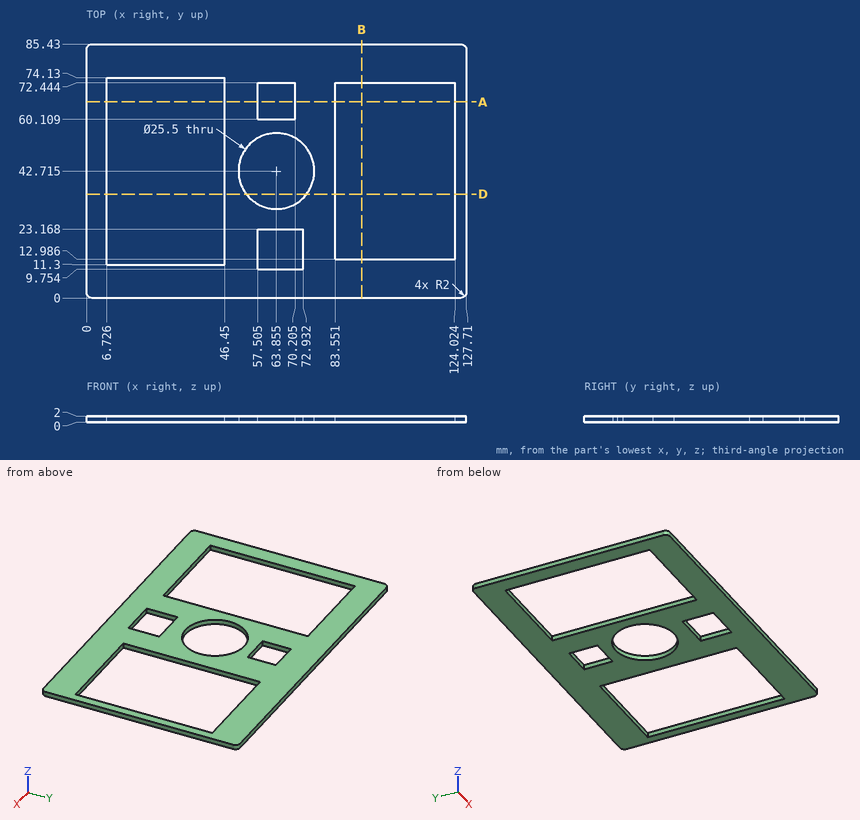
Geometry: see drawing. Coordinates: mm, zero at the bounding-box minimum. Coordinates: 2 decimals unless noted, no trailing zeros. Loops run counter-clockwise (first coordinate to the right, second up) from the corner with the lowest first, then second, coordinate; pieces in that order, holes last. Notation, with made-up numbers: (-39.5, 49.5) - (7.5, 49.5) arc R11 cw to (7.5, 59.5) - close; hole circle Ø7 at (-29, -18). An arc over 180 degrees is marked (long way). Answer in a Markdown table with one row per item.
(1) Material intervals for L1, parallel to X at y = 28, z = 1.7; L2, parallel to Y at x = 64, z = 1.65; L3, parallel to Y at x = 63, z = 1.15, sorted ascending. Write a range as from..to.
Model answer:
| item | result |
|---|---|
| L1 | x = 0..6.73, 46.45..83.55, 124.02..127.71 |
| L2 | y = 0..9.75, 23.17..29.97, 55.46..60.11, 72.44..85.43 |
| L3 | y = 0..9.75, 23.17..29.99, 55.44..60.11, 72.44..85.43 |
(2) Cut plane A-A on y = 66. Count the separate pieces of the cut face and the enclosed holes in it.
Model answer:
| item | result |
|---|---|
| separate pieces | 4 |
| enclosed holes | 0 |
(3) Cut plane D-D on y = 35. Output: boundary loops of the cut face in (x, z).
Model answer:
| item | result |
|---|---|
| outline | (0, 0) - (6.73, 0) - (6.73, 2) - (0, 2) - close; (46.45, 0) - (53.7, 0) - (53.7, 2) - (46.45, 2) - close; (74.01, 0) - (83.55, 0) - (83.55, 2) - (74.01, 2) - close; (124.02, 0) - (127.71, 0) - (127.71, 2) - (124.02, 2) - close |
(4) Cut plane B-B on x = 92.5. Output: boundary loops of the cut face in (y, z).
Model answer:
| item | result |
|---|---|
| outline | (0, 0) - (12.99, 0) - (12.99, 2) - (0, 2) - close; (72.44, 0) - (85.43, 0) - (85.43, 2) - (72.44, 2) - close |
